Design review of the part built by this model. Coordinates are the model's own, in mm. Face numbers are marked on the shaded views. A direction names the side the tool comes from. Give positions to 0.01 mm unless a question says otherwise; leave off trailing zeros. Loops run counter-clockwise (first coordinate to the right, second up) from the corner with the lowest first, then second, coordinate; pieces in that order, holes last. Notation, with made-up numbers: (78, 75.5) -> (84, 75.5) arc R15 cw to (84, 98.5) -> close; hole circle Ø5 at (46.25, 12.5). An arc over 180 degrees is marked (long way). Answer in a Markdown table with one row per item. Add a question column.
(1) Consider section C-C on x = -4. Write out the cut boundary in (y, z), then the cut area to 3 significant figures.
(2) Consider section B-B on y = -25.5. Write out the cut boundary in (x, z).
(3) Draft analysis for pull direction X (two halves, no side actions). For the marked faces 1, 2 and 3, state which applies: +X half, -X half, draft (parallel to the pull), parting line (faces both ways), or undercut.
(4) For line 1 (X direction, y = -67.5, z = 8.5); line 2 (Z direction, x = 8, y = -59.5); line 3 (Y direction, x = -2, z = 82), list the stretches that pass through material, from the lowest coordinate up.
(5) Consider section D-D on y = -75. Write out the cut boundary in (x, z), then the cut area to 3 significant figures.
(6) For pin 1 (10 mm diameter, centred on y = -79.5, z = 20, fed in from +X); pin 2 (12 mm diameter, centred on x = 39.5, z = 46.5, fed in from -Y); pin 3 (13 mm diameter, centred on x = 53.5, y = -23.5, fed in from -Z); pin 4 (0.5 mm diameter, centred on x = -5, y = -40.5, fed in from -Z), all flat-tipped, find the tip position at first contact; note any pin that passes through.
(7) Consider section A-A on z = 18.5. Write out the cut boundary in (x, y), then the cut area to 3 significant figures.
(8) For the marked faces 4, 5 and 6, list the 3-axis set-ups (+Z, -Z, +X, -X, +Y, -Y) from which the entire face can be reached by the end or side of a thin tool; tool diameter is ignored.
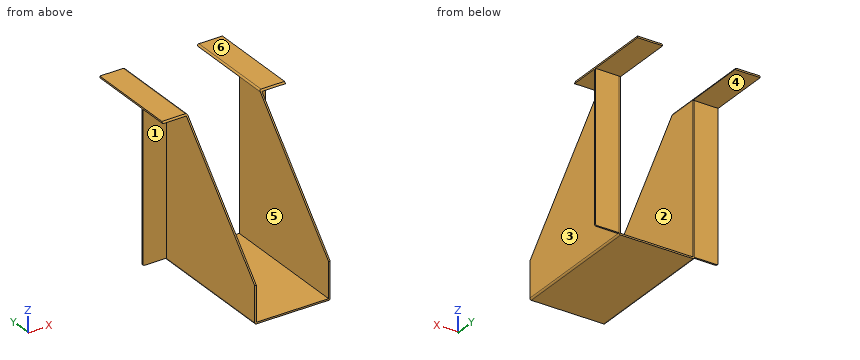
from build123d import *

# Parameters (mm, degrees)
F1_DEPTH      = 125
F2_W          = 45.333487
F2_H          = 99.635656
F3_DEPTH      = 100
F3_DEPTH_BACK = 50
F5_DEPTH      = 1


with BuildPart() as f1:
    # F0 (on Front) → F1 (new body)
    with BuildSketch(Plane.XZ):
        with BuildLine():
            ThreePointArc((0, 1), (0.292893, 0.292893), (1, 0))
            Line((1, 0), (47, 0))
            ThreePointArc((47, 0), (47.707107, 0.292893), (48, 1))
            Line((48, 1), (48, 96))
            Line((48, 96), (63, 96))
            Line((63, 96), (63, 97))
            Line((63, 97), (48, 97))
            ThreePointArc((48, 97), (47.292893, 96.707107), (47, 96))
            Line((47, 96), (47, 1))
            Line((47, 1), (1, 1))
            Line((1, 1), (1, 96))
            ThreePointArc((1, 96), (0.707107, 96.707107), (0, 97))
            Line((0, 97), (-15, 97))
            Line((-15, 97), (-15, 96))
            Line((-15, 96), (0, 96))
            Line((0, 96), (0, 1))
        make_face()
    extrude(amount=F1_DEPTH)

    # F2 (on face) → F3 (cut, two sides)
    with BuildSketch(Plane.YZ.offset(63)) as f3_sk:
        with Locations((-17.320754, 46.182172)):
            Rectangle(F2_W, F2_H)
        Polygon((-139.87067, 100.481688), (-139.87067, 6.786287), (-55.961391, 100.481688), align=None)
    extrude(amount=-F3_DEPTH, mode=Mode.SUBTRACT)
    extrude(f3_sk.sketch, amount=-F3_DEPTH_BACK, mode=Mode.SUBTRACT)

    # F4 (on face) → F5 (join)
    with BuildSketch(Plane(origin=(0, -39.987498, 0), x_dir=(-1, 0, 0), z_dir=(0, 1, 0))):
        with BuildLine():
            Line((-47, 1.063345), (-47, 96))
            Line((-47, 96), (-63, 96))
            Line((-63, 96), (-63, 2.063345))
            ThreePointArc((-63, 2.063345), (-62.707107, 1.356238), (-62, 1.063345))
            Line((-62, 1.063345), (-47, 1.063345))
        make_face()
        with BuildLine():
            Line((15, 2.063345), (15, 96))
            Line((15, 96), (-1, 96))
            Line((-1, 96), (-1, 1.063345))
            Line((-1, 1.063345), (14, 1.063345))
            ThreePointArc((14, 1.063345), (14.707107, 1.356238), (15, 2.063345))
        make_face()
    extrude(amount=-F5_DEPTH)


solid = f1.part
Values follow:
| question | item | result |
|---|---|---|
| 1 | outline | (-59.97, 96) -> (-40.99, 96) -> (-40.99, 1.06) -> (-39.99, 1.06) -> (-39.99, 96) -> (0, 96) -> (0, 97) -> (-59.08, 97) -> close |
| 1 | area | 154 mm2 |
| 2 | outline | (-15, 96) -> (1, 96) arc R1 ccw to (0, 97) -> (-15, 97) -> close; (47, 96) -> (63, 96) -> (63, 97) -> (48, 97) arc R1 ccw to start |
| 3 | face 1 | draft |
| 3 | face 2 | undercut |
| 3 | face 3 | +X half |
| 4 | line 1 | 0 to 1, 47 to 48 |
| 4 | line 2 | 0 to 1 |
| 4 | line 3 | -40.99 to -39.99 |
| 5 | outline | (0, 1) arc R1 ccw to (1, 0) -> (47, 0) arc R1 ccw to (48, 1) -> (48, 79.22) -> (47, 79.22) -> (47, 1) -> (1, 1) -> (1, 79.22) -> (0, 79.22) -> close |
| 5 | area | 204 mm2 |
| 6 | pin 1 | x = 48 |
| 6 | pin 2 | through |
| 6 | pin 3 | z = 96 |
| 6 | pin 4 | z = 1.06 |
| 7 | outline | (-15, -40.99) -> (0, -40.99) -> (0, -125) -> (1, -125) -> (1, -39.99) -> (-15, -39.99) -> close; (47, -125) -> (48, -125) -> (48, -40.99) -> (63, -40.99) -> (63, -39.99) -> (47, -39.99) -> close |
| 7 | area | 200 mm2 |
| 8 | face 4 | -Z, +X, -X, +Y |
| 8 | face 5 | +Z, +Y, -Y |
| 8 | face 6 | +Z, +X, -X, +Y, -Y |
